Geometry: final body of the model. Coordinates: model frame, mm. A direction names the side the tool comes from. Coordinates: 2 decimals unless noted, no trailing zeros. Order: outer loops, then holes, each group sorted by start corner. A loop starts at its lowest first (then second) coordinate and runs counter-clockwise, first axis right, second up. Notation, with made-up numbers: M 29,-12 L 79,-12 A22 ccw 79,13 Z; hole C 49.5,88 d2. An arc over 180 degrees is marked long. Use CSV: the item, a comma, the result in double quotes. Start each with the question number.
1. Material intervals for line 1 (Z direction, x = 0, y = 0.35); line 2 (X direction, y = 1.35, z = 8.25); line 3 (X direction, y = -0.1, z = -7.5), sorted ascending.
2. Pull-direction query (X, two-part tool) for faces 6 (the flat face through (4.17, 0, 0)), 7 (the cylindrical face through (-4.75, -0.02, -5.02)), 8 (the cylindrical face through (-4.954, -0.021, 1.943)), 9 (the flat face through (-6, -1.5, -3)); classes: pulls with the +X half, pulls with the -X half, needs draft (parallel to the pull), parting line crosses it, or undercut.
3. Section query A-A on x = 0. Return the cut outline in (y, z), and give its area (3 significant figures).
4. First-contact query: P1, Ø0.9, axis at y = 0, z = 8, coming from the +X side; P2, Ø0.9, axis at x = -2.5, y = 0.5, coming from the +Z side; P3, Ø1, axis at y = -0.5, z = -5, coming from the -X side; P4, Ø2, axis at x = -17.16, z = -10, coming from the -Y side (3 decimals). Flat tips, straight axial feed; report the tip coordinate or a pass-through.
5. Set-up query: faces 1 (the cylindrical face through (-17.828, -0.021, -11.054)), 2 (the flat face through (-3, 0, 6.056)), 3 (the flat face through (0, 0, -11.944)), 4 (the flat face through (3, 0, 6.056)), 5 (the flat face through (-1.23, 0, -9)). Return all of +Z, -Z, +X, -X, +Y, -Y with unobstructed straight access to the full face (end or side cutting, diameter ignored); none if empty.
6. Section query D-D on x = -13.75. Return the cut outline in (y, z).
7. Section query C-C on z = 2.5. Return the cut outline in (x, y), and give its area (3 significant figures).
8. Section query B-B on y = -0.75. State how many separate pieces and enclosed holes the cut face has, and give its area (3 significant figures).
Autodesk Inventor part; units mm, degrees
ref_plane "YZ Plane" through (0, 0, 0) normal (1, 0, 0) x (0, 1, 0)
ref_plane "XZ Plane" through (0, 0, 0) normal (0, 1, 0) x (-1, 0, 0)
ref_plane "XY Plane" through (0, 0, 0) normal (0, 0, 1) x (1, 0, 0)
sketch "草圖1" plane through (0, 0, 0) normal (0, 1, 0) x (-1, 0, 0)
  line L0 (4.2304, -5.8965) -> (4.2304, -5.9439)
  line L1 (4.2304, -5.9439) -> (0.0304, -5.9439)
  line L2 (0.0304, -5.9439) -> (1.2304, -5.9439)
  line L3 (1.2304, -5.9439) -> (1.2304, -11.9439)
  line L4 (1.2304, -11.9439) -> (0.0304, -11.9439)
  line L5 (-4.1696, 0.0561) -> (-4.1696, -5.9439)
  line L6 (-4.1696, -5.9439) -> (0.0304, -5.9439)
  line L7 (0.0304, -5.9439) -> (-1.1696, -5.9439)
  line L8 (-1.1696, -5.9439) -> (-1.1696, -11.9439)
  line L9 (-1.1696, -11.9439) -> (0.0304, -11.9439)
  line L10 (4.2304, 4.5332) -> (4.2304, 6.0561)
  line L11 (4.2304, 6.0561) -> (0.0304, 6.0561)
  line L12 (0.0304, 6.0561) -> (1.2304, 6.0561)
  line L13 (1.2304, 6.0561) -> (1.2304, 12.0561)
  line L14 (1.2304, 12.0561) -> (0.0304, 12.0561)
  line L15 (-4.1696, 0.0561) -> (-4.1696, 6.0561)
  line L16 (-4.1696, 6.0561) -> (0.0304, 6.0561)
  line L17 (0.0304, 6.0561) -> (-1.1696, 6.0561)
  line L18 (-1.1696, 6.0561) -> (-1.1696, 12.0561)
  line L19 (-1.1696, 12.0561) -> (0.0304, 12.0561)
  circle A0 centre (0, 0) radius 1.5
  circle A1 centre (17.1565, -10) radius 1.25
  arc A2 (13.2007, -10.5927) -> (19.0627, -6.4834) centre (17.1565, -10) ccw
  line L20 (19.0627, -6.4834) -> (6.8478, 0.1374)
  line L21 (12.7818, -9.9193) -> (5.8005, -5.075)
  arc A3 (4.2304, 4.5332) -> (6.8478, 0.1374) centre (9.2304, 4.5332) ccw
  arc A4 (5.8005, -5.075) -> (4.2304, -5.8965) centre (5.2304, -5.8965) ccw
  arc A5 (13.2007, -10.5927) -> (12.7818, -9.9193) centre (12.2117, -10.7409) ccw
  point P0 (4.2304, 0.0561)
  point P1 (13.1607, -10.1822)
  dimension "d0" = 6
  dimension "d1" = 1.2
  dimension "d2" = 3
  dimension "d3" = 6
  dimension "d4" = 3
  dimension "d9" = 2.5
  dimension "d10" = 8
  dimension "d11" = 5
  dimension "d12" = 1
  dimension "d13" = 1
extrude "擠出1" add sketch "草圖1" along normal mid plane 3
properties part number "小零件3"
Results list:
1,line 1,"z = -11.94 to -1.5, 1.5 to 12.06"
1,line 2,"x = -1.23 to 1.17"
1,line 3,"x = -20.28 to -9.3, -1.23 to 1.17"
2,face 6,"pulls with the +X half"
2,face 7,"undercut"
2,face 8,"pulls with the -X half"
2,face 9,"needs draft"
3,outline,"M -1.5,-11.94 L 1.5,-11.94 L 1.5,-1.5 L -1.5,-1.5 Z; M -1.5,1.5 L 1.5,1.5 L 1.5,12.06 L -1.5,12.06 Z"
3,area,"63.0 mm²"
4,P1,"stops at x = 1.17"
4,P2,"stops at z = 6.06"
4,P3,"stops at x = -17.25"
4,P4,"passes through"
5,face 1,"+Y, -Y"
5,face 2,"+Z, -X, +Y, -Y"
5,face 3,"-Z, +X, +Y, -Y"
5,face 4,"+Z, +X, +Y, -Y"
5,face 5,"-Z, +Y, -Y"
6,outline,"M -1.5,-12.1 L 1.5,-12.1 L 1.5,-3.6 L -1.5,-3.6 Z"
7,outline,"M -4.66,-1.5 L 4.17,-1.5 L 4.17,1.5 L -4.66,1.5 Z"
7,area,"26.5 mm²"
8,separate pieces,"1"
8,enclosed holes,"2"
8,area,"236 mm²"
